Here's how the part is built. I have some questions about the finished solid (model axes, mm). A direction names the side the tool comes from. Round coordinates to 2 decimals unless told otherwise and drop trailing zeros. Loops run counter-clockwise (first coordinate to the right, second up) from the corner with the lowest first, then second, coordinate; pieces in that order, holes last. Notation, with made-up numbers: M 81,67 L 116,67 A22 cw 116,79 Z; hole C 51.5,38.25 d2. An arc over 180 degrees is marked long. Answer as CSV lines item,"result".
```python
from build123d import *

# Parameters (mm, degrees)
PAD_DEPTH    = 40
SKETCH001_R  = 4.1
POCKET_DEPTH = 70.0155982259


with BuildPart() as part:
    # Sketch (on XY_Plane of Origin) → Pad (new body)
    with BuildSketch(Plane.XY):
        Polygon((-35, 0), (-35, 110), (-35, 152.37407), (-20, 152.37407), (-20, 200), (0, 200), (20.001688, 200), (20.001688, 152.37407), (35.001688, 152.37407), (35.0001418741, 107.5269458609), (34.9829445099, -2.4730527948), (19.9829445099, -2.4730527948), (20.0008612126, 127.5269459706), (0, 127.5269459706), (-20, 127.5269459706), (-20, 0), align=None)
    extrude(amount=PAD_DEPTH)

    # Sketch001 (on Face3 of Pad) → Pocket (cut, through all)
    with BuildSketch(Plane(origin=(34.9833302911, -0.0054692826, 0), x_dir=(0.0001563397, 0.9999999878, 0), z_dir=(0.9999999878, -0.0001563397, 0))):
        with Locations((12.5324164576, 20)):
            Circle(SKETCH001_R)
    extrude(amount=-POCKET_DEPTH, mode=Mode.SUBTRACT)


solid = part.part
```
1. We'd pull the mould along Z, two halves only. Please class faces 5 (the flat face through (20.002, 177, 20)), 6 (the flat face through (-23, 100, 40)), 7 (the cylindrical face through (-27.4, 9.28, 17.51)): pulls with the +Z half, pulls with the -Z half, needs draft (parallel to the pull), parting line crosses it, or undercut.
Evaluation:
face 5,"needs draft"
face 6,"pulls with the +Z half"
face 7,"undercut"
2. If I drill on line 1 (X direction, y = 33, z = 24.5); line 2 (Y direction, x = -29, z = 20); line 3 (Y direction, x = 24.75, z = 20), over which ranges is the centre line in solid material (lowest first)? Write a range as [from, to].
Evaluation:
line 1,"x = [-35, -20], [19.99, 34.99]"
line 2,"y = [0, 8.44], [16.64, 152.37]"
line 3,"y = [-2.47, 8.43], [16.63, 152.37]"
3. I want a section at A-A, the plane z = 22. Please give me the cut outline in (x, y).
Evaluation:
outline,"M -35,0 L -20,0 L -20,8.96 L -35,8.96 Z; M -35,16.12 L -20,16.11 L -20,127.53 L 20,127.53 L 19.99,16.11 L 34.99,16.11 L 35,107.53 L 35,152.37 L 20,152.37 L 20,200 L -20,200 L -20,152.37 L -35,152.37 Z; M 19.98,-2.47 L 34.98,-2.47 L 34.98,8.95 L 19.98,8.95 Z"
4. I want a section at C-C, the plane z = 35. Please give me the cut outline in (x, y).
Evaluation:
outline,"M -35,0 L -20,0 L -20,127.53 L 20,127.53 L 19.98,-2.47 L 34.98,-2.47 L 35,107.53 L 35,152.37 L 20,152.37 L 20,200 L -20,200 L -20,152.37 L -35,152.37 Z"
5. For P1, Ø10, axis at x = 1, z = 12, coming from the -Y side; P2, Ø5, axis at y = 12.53, z = 20, coming from the -X side; P3, Ø1.5, axis at y = 89, z = 11.5, coming from the +X side; P4, Ø12, axis at y = 173.5, z = 27.5, coming from the -X side, each with a flat end and sliding along its axis, tell me the tip position at first contact or that it passes through.
Evaluation:
P1,"stops at y = 127.53"
P2,"passes through"
P3,"stops at x = 35"
P4,"stops at x = -20"
6. Which directions (+Z, -Z, +X, -X, +Y, -Y) give clear straight access to the entire face, cutting with the end or side of a thin tool? Please do faces 1 (the flat face through (27, 152.374, 20)), 2 (the flat face through (-27, 0, 20)), 3 (the flat face through (-20, 176, 20)), 4 (the flat face through (-20, 65, 20)).
Evaluation:
face 1,"+Z, -Z, +X, +Y"
face 2,"+Z, -Z, -X, -Y"
face 3,"+Z, -Z, -X, +Y"
face 4,"+Z, -Z, -Y"
7. I want a section at B-B, the plane y = 33. Please give me the cut outline in (x, z).
Evaluation:
outline,"M -35,0 L -20,0 L -20,40 L -35,40 Z; M 19.99,0 L 34.99,0 L 34.99,40 L 19.99,40 Z"
8. I want a section at D-D, the plane y = 116.5. Please give me the cut outline in (x, z).
Evaluation:
outline,"M -35,0 L -20,0 L -20,40 L -35,40 Z; M 20,0 L 35,0 L 35,40 L 20,40 Z"
